Read the model definition and answer for the solid it produces. Units are mm, in the model's axes. A direction names the side the tool comes from. Coordinates: 2 decimals unless noted, no trailing zeros. Order: outer loops, then holes, each group sorted by start corner. A loop starts at its lowest first (then second) coordinate and runs counter-clockwise, first axis right, second up. Notation, with made-up numbers: (73, 21) -> (100, 21) arc R31 ccw to (100, 57) -> close; hole circle Ø11 at (49, 80). An arc over 180 degrees is marked (long way). Use CSV: the item, a comma, the result in double quotes.
```python
from build123d import *

# Parameters (mm, degrees)
SKETCH1_W            = 30.000000000000004
SKETCH1_H            = 30.000000000000004
BOSS_EXTRUDE3_DEPTH  = 12
SKETCH2_W            = 26.999999999999993
SKETCH2_H            = 27.000000000000007
CUT_EXTRUDE1_DEPTH   = 10
FILLET1_START        = -1
FILLET1_DEPTH        = 13
FILLET1_START_2      = 1.13256
FILLET1_2_DEPTH      = 10.86744
CUT_EXTRUDE2_DEPTH   = 2.5
CUT_EXTRUDE2_DRAFT   = 1.0000000000000042
MIRROR1_COPY_1_DEPTH = 2.5
MIRROR1_COPY_1_DRAFT = 1.0000000000000042
CUT_EXTRUDE3_DEPTH   = 7.62
SKETCH6_R            = 2.6750000000000007
BOSS_EXTRUDE4_DEPTH  = 6
SKETCH6_2_R          = 2.6750000000000007
BOSS_EXTRUDE5_DEPTH  = 0.5
CUT_EXTRUDE4_REACH   = 26.372
FILLET2_SIZE         = 1


with BuildPart() as part:
    # Sketch1 → Boss-Extrude3 (new body)
    with BuildSketch(Plane(origin=(0, 0, 0), x_dir=(1, 0, 0), z_dir=(0, 1, 0))):
        Rectangle(SKETCH1_W, SKETCH1_H)
    extrude(amount=BOSS_EXTRUDE3_DEPTH)

    # Sketch2 → Cut-Extrude1 (cut)
    with BuildSketch(Plane(origin=(0, 12, 0), x_dir=(1, 0, 0), z_dir=(0, 1, 0))):
        Rectangle(SKETCH2_W, SKETCH2_H)
    extrude(amount=-CUT_EXTRUDE1_DEPTH, mode=Mode.SUBTRACT)

    # Fillet1: read off the stored shape, not the designer's step
    # Fillet1 outline → Fillet1 (cut)
    with BuildSketch(Plane(origin=(0, 0, 0), x_dir=(1, 0, 0), z_dir=(0, 1, 0)).offset(FILLET1_START)):
        with BuildLine():
            Line((-8.55, 15), (8.55, 15))
            add(Edge.make_bspline(
                [(8.55, 15), (9.63487743239395, 15), (10.7197548647879, 15), (13.1108387386532, 14.5375871170573), (14.5375871170573, 13.1108387386532), (15, 10.7197548647879), (15, 9.63487743239395), (15, 8.55)],
                knots=[0, 0, 0, 0, 0, 0, 0.5, 0.5, 1, 1, 1, 1, 1, 1], degree=5))
            Line((15, 8.55), (15, 7))
            Line((15, 7), (17, 7))
            Line((17, 7), (17, 17))
            Line((17, 17), (-17, 17))
            Line((-17, 17), (-17, 7))
            Line((-17, 7), (-15, 7))
            Line((-15, 7), (-15, 8.55))
            add(Edge.make_bspline(
                [(-15, 8.55), (-15, 9.63487743239395), (-15, 10.7197548647879), (-14.5375871170573, 13.1108387386532), (-13.1108387386532, 14.5375871170573), (-10.7197548647879, 15), (-9.63487743239395, 15), (-8.55, 15)],
                knots=[0, 0, 0, 0, 0, 0, 0.5, 0.5, 1, 1, 1, 1, 1, 1], degree=5))
        make_face()
    extrude(amount=FILLET1_DEPTH, mode=Mode.SUBTRACT)

    # Fillet1 2 outline → Fillet1 2 (add)
    with BuildSketch(Plane(origin=(0, 0, 0), x_dir=(1, 0, 0), z_dir=(0, 1, 0)).offset(FILLET1_START_2)):
        with BuildLine():
            add(Edge.make_bspline(
                [(8.55, 15), (9.63487743239395, 15), (10.7197548647879, 15), (13.1108387386532, 14.5375871170573), (14.5375871170573, 13.1108387386532), (15, 10.7197548647879), (15, 9.63487743239395), (15, 8.55)],
                knots=[0, 0, 0, 0, 0, 0, 0.5, 0.5, 1, 1, 1, 1, 1, 1], degree=5))
            Line((8.55, 15), (-8.55, 15))
            add(Edge.make_bspline(
                [(-15, 8.55), (-15, 9.63487743239395), (-15, 10.7197548647879), (-14.5375871170573, 13.1108387386532), (-13.1108387386532, 14.5375871170573), (-10.7197548647879, 15), (-9.63487743239395, 15), (-8.55, 15)],
                knots=[0, 0, 0, 0, 0, 0, 0.5, 0.5, 1, 1, 1, 1, 1, 1], degree=5))
            Line((-15, 8.55), (-15, 7))
            Line((-15, 7), (-13.5, 7))
            Line((-13.5, 7), (-13.5, 9.5))
            add(Edge.make_bspline(
                [(-9.5, 13.5), (-10.1727922061358, 13.5), (-10.8455844122716, 13.5), (-12.3284271247462, 13.2132323206557), (-13.2132323206557, 12.3284271247462), (-13.5, 10.8455844122716), (-13.5, 10.1727922061358), (-13.5, 9.5)],
                knots=[0, 0, 0, 0, 0, 0, 0.5, 0.5, 1, 1, 1, 1, 1, 1], degree=5))
            Line((-9.5, 13.5), (9.5, 13.5))
            add(Edge.make_bspline(
                [(13.5, 9.5), (13.5, 10.1727922061358), (13.5, 10.8455844122716), (13.2132323206557, 12.3284271247462), (12.3284271247462, 13.2132323206557), (10.8455844122716, 13.5), (10.1727922061358, 13.5), (9.5, 13.5)],
                knots=[0, 0, 0, 0, 0, 0, 0.5, 0.5, 1, 1, 1, 1, 1, 1], degree=5))
            Line((13.5, 9.5), (13.5, 7))
            Line((13.5, 7), (15, 7))
            Line((15, 7), (15, 8.55))
        make_face()
    extrude(amount=FILLET1_2_DEPTH)


with BuildPart() as cut_extrude2_tool:
    # Sketch3 → Cut-Extrude2 (with draft: the straight prism first)
    with BuildSketch(Plane(origin=(0, 12, 0), x_dir=(1, 0, 0), z_dir=(0, 1, 0))):
        Polygon((-15.000000000000002, 8.040000000000003), (-14.999999999999998, -7.959999999999998), (-13.499999999999986, -7.959999999999998), (-13.499999999999988, 8.040000000000003), align=None)
    extrude(amount=-CUT_EXTRUDE2_DEPTH)
    # Cut-Extrude2: the draft: its side faces are tilted about the plane it starts from
    cut_extrude2_sides = [cut_extrude2_tool.faces().sort_by_distance(p)[0] for p in [
        (-15, 10.75, -0.04),
        (-14.25, 10.75, 7.96),
        (-13.5, 10.75, -0.04),
        (-14.25, 10.75, -8.04),
    ]]
    draft(cut_extrude2_sides, Plane(origin=(0, 12, 0), x_dir=(1, 0, 0), z_dir=(0, 1, 0)), CUT_EXTRUDE2_DRAFT)


with BuildPart() as part_1:
    add(part.part)

    # Cut-Extrude2: cut by cut_extrude2_tool
    add(cut_extrude2_tool.part, mode=Mode.SUBTRACT)


with BuildPart() as mirror1_copy_1_tool:
    # Mirror1 copy 1 sketch → Mirror1 copy 1 (with draft: the straight prism first)
    with BuildSketch(Plane(origin=(0, 12, 0), x_dir=(-1, 0, 0), z_dir=(0, 1, 0))):
        Polygon((-15.000000000000002, -8.040000000000003), (-14.999999999999998, 7.959999999999998), (-13.499999999999986, 7.959999999999998), (-13.499999999999988, -8.040000000000003), align=None)
    extrude(amount=-MIRROR1_COPY_1_DEPTH)
    # Mirror1 copy 1: the draft: its side faces are tilted about the plane it starts from
    mirror1_copy_1_sides = [mirror1_copy_1_tool.faces().sort_by_distance(p)[0] for p in [
        (15, 10.75, -0.04),
        (14.25, 10.75, 7.96),
        (13.5, 10.75, -0.04),
        (14.25, 10.75, -8.04),
    ]]
    draft(mirror1_copy_1_sides, Plane(origin=(0, 12, 0), x_dir=(-1, 0, 0), z_dir=(0, 1, 0)), MIRROR1_COPY_1_DRAFT)


with BuildPart() as part_2:
    add(part_1.part)

    # Mirror1 copy 1: cut by mirror1_copy_1_tool
    add(mirror1_copy_1_tool.part, mode=Mode.SUBTRACT)

    # Sketch5 → Cut-Extrude3 (cut)
    with BuildSketch(Plane(origin=(0, 12, 0), x_dir=(1, 0, 0), z_dir=(0, 1, 0))):
        Polygon((-10.006699639770744, -14.999999999999998), (10.006699639770742, -14.999999999999998), (10.006699639770742, -13.5), (-10.006699639770742, -13.500000000000002), align=None)
    extrude(amount=-CUT_EXTRUDE3_DEPTH, mode=Mode.SUBTRACT)

    # Sketch6 → Boss-Extrude4 (add)
    # profile 1 of 2: a face of its own
    with BuildSketch(Plane(origin=(0, 2, 0), x_dir=(1, 0, 0), z_dir=(0, 1, 0))):
        with BuildLine():
            Line((10.49999999999986, -6.5), (13.5, -6.5))
            Line((13.5, -6.5), (13.5, 0.5000000000000004))
            Line((13.5, 0.5000000000000004), (10.49999999999986, 0.5000000000000004))
            ThreePointArc((10.49999999999986, 0.5000000000000004), (6.99999999999986, -3), (10.49999999999986, -6.5))
        make_face()
        with Locations(Location((10.49999999999986, -2.9999999999999996, 0), (0, 0, 270))):
            Circle(SKETCH6_R, mode=Mode.SUBTRACT)
    # profile 2 of 2: a face of its own
    with BuildSketch(Plane(origin=(0, 2, 0), x_dir=(1, 0, 0), z_dir=(0, 1, 0))):
        Polygon((13.5, 9.500000000000004), (13.5, 6.0000000000000036), (7, 6.000000000000003), (7, 13.500000000000004), (13.5, 13.500000000000004), align=None)
        with Locations(Location((10.49999999999986, 9.5, 0), (0, 0, 270))):
            Circle(SKETCH6_R, mode=Mode.SUBTRACT)
    boss_extrude4 = extrude(amount=BOSS_EXTRUDE4_DEPTH)

    # Sketch6<2> → Boss-Extrude5 (add)
    with BuildSketch(Plane(origin=(0, 2, 0), x_dir=(1, 0, 0), z_dir=(0, 1, 0))):
        with Locations(Location((10.49999999999986, 9.5, 0), (0, 0, 270))):
            Circle(SKETCH6_2_R)
        with Locations(Location((10.49999999999986, -2.9999999999999996, 0), (0, 0, 270))):
            Circle(SKETCH6_2_R)
    boss_extrude5 = extrude(amount=BOSS_EXTRUDE5_DEPTH)

    # Cut-Extrude4: up to this face of the body (flat: up to its plane)
    cut_extrude4_end = Plane(part_2.part.faces().sort_by_distance((-14.25, 9.5, -0.04))[0])
    # Sketch13 → Cut-Extrude4 (cut, up to the picked face)
    with BuildSketch(Plane(origin=(0, 0, 0), x_dir=(-1, 0, 0), z_dir=(0, -1, 0)), mode=Mode.PRIVATE) as cut_extrude4_sk1:
        Polygon((14.999999999999998, -7.99636233767945), (14.499999999999996, -7.99636233767945), (14.5, 8.083637662320546), (15, 8.083637662320546), align=None)
    cut_extrude4_tool1 = split(extrude(cut_extrude4_sk1.sketch, amount=-CUT_EXTRUDE4_REACH, mode=Mode.PRIVATE), bisect_by=cut_extrude4_end, keep=Keep.BOTH, mode=Mode.PRIVATE)
    cut_extrude4 = cut_extrude4_tool1.solids().sort_by(Axis((-14.75, 0, -0.043638), (0, 1, 0)))[0]
    add(cut_extrude4, mode=Mode.SUBTRACT)

    # Mirror2: Boss-Extrude4, Boss-Extrude5, Cut-Extrude4 across plane
    add(boss_extrude4.mirror(Plane.ZY))
    add(boss_extrude5.mirror(Plane.ZY))
    add(cut_extrude4.mirror(Plane.ZY), mode=Mode.SUBTRACT)

    # Fillet2
    # a fillet whose section is not a circle: 1 mm, written as the material it takes off along each edge
    with BuildSketch(Plane(origin=(-7, 2, -6.000000000000003), x_dir=(-1, 0, 0), z_dir=(0, 1, 0))) as fillet2_piece_1:
        with BuildLine():
            add(Edge.make_bspline([(FILLET2_SIZE, 0), (FILLET2_SIZE * 0.831801948466, 0), (FILLET2_SIZE * 0.663603896932, 0), (FILLET2_SIZE * 0.292893218813, -FILLET2_SIZE * 0.0716919198361), (FILLET2_SIZE * 0.0716919198361, -FILLET2_SIZE * 0.292893218813), (0, -FILLET2_SIZE * 0.663603896932), (0, -FILLET2_SIZE * 0.831801948466), (0, -FILLET2_SIZE)], knots=[0, 0, 0, 0, 0, 0, 0.5, 0.5, 1, 1, 1, 1, 1, 1], degree=5))
            Line((0, -FILLET2_SIZE), (0, 0))
            Line((0, 0), (FILLET2_SIZE, 0))
        make_face()
    extrude(amount=8.5, mode=Mode.SUBTRACT)
    with BuildSketch(Plane(origin=(7, 2, -6.000000000000003), x_dir=(1, 0, 0), z_dir=(0, 1, 0))) as fillet2_piece_2:
        with BuildLine():
            add(Edge.make_bspline([(FILLET2_SIZE, 0), (FILLET2_SIZE * 0.831801948466, 0), (FILLET2_SIZE * 0.663603896932, 0), (FILLET2_SIZE * 0.292893218813, FILLET2_SIZE * 0.0716919198361), (FILLET2_SIZE * 0.0716919198361, FILLET2_SIZE * 0.292893218813), (0, FILLET2_SIZE * 0.663603896932), (0, FILLET2_SIZE * 0.831801948466), (0, FILLET2_SIZE)], knots=[0, 0, 0, 0, 0, 0, 0.5, 0.5, 1, 1, 1, 1, 1, 1], degree=5))
            Line((0, FILLET2_SIZE), (0, 0))
            Line((0, 0), (FILLET2_SIZE, 0))
        make_face()
    extrude(amount=8.5, mode=Mode.SUBTRACT)

    # Sketch9 → Revolve1 (revolve)
    with BuildSketch(Plane(origin=(-12.240866923994627, 8, -7.468988588672871), x_dir=(-0.6507913734559867, 0, 0.7592566023652811), z_dir=(-0.7592566023652811, 0, -0.6507913734559867)), mode=Mode.PRIVATE) as revolve1_sk:
        with BuildLine():
            Line((0, -1), (0, 0))
            ThreePointArc((0, 0), (-0.17693514578671132, -0.4999999999999999), (0, -1))
        make_face()
    revolve(revolve1_sk.sketch.rotate(Axis((-10.49999999999986, 19.424716620639604, -9.5), (0, -1, 0)), 319.398705355), axis=Axis((-10.49999999999986, 19.424716620639604, -9.5), (0, -1, 0)))

    # Sketch10 → Revolve2 (revolve)
    with BuildSketch(Plane(origin=(12.240866923994627, 8, -7.468988588672871), x_dir=(-0.6507913734559867, 0, -0.7592566023652811), z_dir=(0.7592566023652811, 0, -0.6507913734559867)), mode=Mode.PRIVATE) as revolve2_sk:
        with BuildLine():
            Line((0, -1), (0, 0))
            ThreePointArc((0, 0), (0.19685183327597433, -0.5), (0, -1))
        make_face()
    revolve(revolve2_sk.sketch.rotate(Axis((10.49999999999986, 19.424716620639604, -9.5), (0, -1, 0)), 40.601294645), axis=Axis((10.49999999999986, 19.424716620639604, -9.5), (0, -1, 0)))

    # Sketch11 → Revolve3 (revolve)
    with BuildSketch(Plane(origin=(-12.240866923994624, 8, 5.031011411327126), x_dir=(-0.650791373455986, 0, 0.7592566023652817), z_dir=(-0.7592566023652816, 0, -0.6507913734559859)), mode=Mode.PRIVATE) as revolve3_sk:
        with BuildLine():
            Line((0, 0), (1.2e-16, -1))
            ThreePointArc((1.2e-16, -1), (-0.20710678118654702, -0.4999999999999998), (0, 0))
        make_face()
    revolve(revolve3_sk.sketch.rotate(Axis((-10.49999999999986, 19.424716620639604, 2.9999999999999996), (0, -1, 0)), 319.398705355), axis=Axis((-10.49999999999986, 19.424716620639604, 2.9999999999999996), (0, -1, 0)))

    # Sketch12 → Revolve4 (revolve)
    with BuildSketch(Plane(origin=(12.240866923994624, 8, 5.031011411327126), x_dir=(-0.650791373455986, 0, -0.7592566023652817), z_dir=(0.7592566023652816, 0, -0.6507913734559859)), mode=Mode.PRIVATE) as revolve4_sk:
        with BuildLine():
            Line((0, -1), (0, 0))
            ThreePointArc((0, 0), (0.16237280325092585, -0.5), (0, -1))
        make_face()
    revolve(revolve4_sk.sketch.rotate(Axis((10.49999999999986, 19.424716620639604, 2.9999999999999996), (0, -1, 0)), 40.601294645), axis=Axis((10.49999999999986, 19.424716620639604, 2.9999999999999996), (0, -1, 0)))


solid = part_2.part
```
Item 1: Each of these flat-tipped pins is pushed along its axis until it touches: P1, Ø0.9, axis at x = -11.5, y = 6.5, coming from the -Z side; P2, Ø5, axis at x = 1.5, z = 4.5, coming from the +Y side; P3, Ø5, axis at x = 2.5, y = 7, coming from the +Z side. Where does it stop, or does it pass through?
Return value:
P1,"stops at z = -14.82"
P2,"stops at y = 2"
P3,"stops at z = -13.5"
Item 2: A tool of negligible diameter and unlimited length cuts with its end or side. For faces 1 (the cylindrical face through (-9.475, 4.719, 5.471)), 2 (the flat face through (0, 0, 0)), 3 (the flat face through (0, 2, 0)), from which of +Z, -Z, +X, -X, +Y, -Y can it reach the whole face along a straight path? Write none if from no direction.
Return value:
face 1,"none"
face 2,"+Z, -Z, +X, -X, -Y"
face 3,"+Y"
Item 3: Find section A-A, the plane x = 2.5. Give the vertices of the cut face in (y, z), then the cut area to 3 significant figures.
Return value:
outline,"(0, -15) -> (12, -15) -> (12, -13.5) -> (2, -13.5) -> (2, 13.5) -> (4.38, 13.5) -> (4.38, 15) -> (0, 15) -> close"
area,"78.6 mm^2"
Item 4: Find section B-B, the plane y = 6. Give the number of separate pieces and of enclosed holes in the cut face, then the cut area to 3 significant figures.
Return value:
separate pieces,"1"
enclosed holes,"4"
area,"202 mm^2"
Item 5: Find section C-C, the plane z = 11.5. Give the vertices of the cut face in (x, y), then the cut area to 3 significant figures.
Return value:
outline,"(-15, 0) -> (15, 0) -> (15, 12) -> (13.5, 12) -> (13.5, 2) -> (-13.5, 2) -> (-13.5, 12) -> (-15, 12) -> close"
area,"90.0 mm^2"
Item 6: Straight lines are drawn through the part: line 1 along X through (y, z) = (3.45, 3) (3 decimals); line 2 along Z through (x, y) = (10.5, 5.45) (3 decimals); line 3 along X through (y, z) = (6.5, 2.5). For each, find the intervals that lie inside material, in ascending order.
Return value:
line 1,"x = -14.5 to -13.175, -7.825 to -7, 7 to 7.825, 13.175 to 14.5"
line 2,"z = -14.912 to -12.175, -6.825 to -6, -0.5 to 0.325, 5.675 to 6.5, 13.5 to 15"
line 3,"x = -14.5 to -13.13, -7.87 to -7.04, 7.04 to 7.87, 13.13 to 14.5"
Item 7: The mould has two halves that part along X. Classify faces 4 (the flat face through (10.007, 8, 14)), 5 (the flat face through (0, 3, 15)), 6 (the flat face through (-14.5, 5, 0)): +X half, -X half, draft (parallel to the pull), parting line (faces both ways), or undercut.
Return value:
face 4,"undercut"
face 5,"draft"
face 6,"-X half"
